Autodesk Inventor part; units mm, degrees
ref_plane "YZ Plane" through (0, 0, 0) normal (1, 0, 0) x (0, 1, 0)
ref_plane "XZ Plane" through (0, 0, 0) normal (0, 1, 0) x (-1, 0, 0)
ref_plane "XY Plane" through (0, 0, 0) normal (0, 0, 1) x (1, 0, 0)
sketch "Skizze1" plane through (0, 0, 0) normal (0, 0, 1) x (1, 0, 0)
  circle A0 centre (0, 0) radius 11
  dimension "d0" = 22
extrude "Extrusion1" add sketch "Skizze1" along normal blind 50.5
sketch "Skizze2" plane through (0, 0, 50.5) normal (0, 0, 1) x (1, 0, 0)
  circle A0 centre (0, 0) radius 3
  circle A1 centre (0, 0) radius 2.5
  circle A2 centre (0, 0) radius 1.5
  dimension "d3" = 6
  dimension "d4" = 5
  dimension "d9" = 3
extrude "Extrusion2" add sketch "Skizze2" along normal blind 1 contours A0 | A1 | A2
extrude "Extrusion3" add sketch "Skizze2" along normal blind 2.5 contours A1 | A2
extrude "Extrusion4" add sketch "Skizze2" along normal blind 11.5 contours A2
properties part number "MotorStanger"
Geometry: final body of the model. Coordinates: model frame, mm. A direction names the side the tool comes from. Round coordinates to 2 decimals unless told otherwise and drop trailing zeros. Order: outer loops, then holes, each group sorted by start corner. A loop starts at its lowest first (then second) coordinate and runs counter-clockwise, first axis right, second up.
Q1. Section C-C, the plane z = 23.5. Output: boundary loops of the cut face in (x, y), and give its area (3 significant figures).
Result sheet:
outline: circle Ø22 at (0, 0)
area: 380 mm2
Q2. Material intervals for probe 1 along Z at (x, y) = (-6, 6.5); probe 2 along Y at (x, z) = (-0.25, 14.5); probe 3 along X at (y, z) = (2.75, 48), sorted ascending.
Result sheet:
probe 1: z = 0 to 50.5
probe 2: y = -11 to 11
probe 3: x = -10.65 to 10.65
Q3. Access query for faces 1 (the face through (-2.38, 10.74, 24.9)), 2 (the face through (-0.54, 2.44, 52.24)). Directions: +Z, -Z, +X, -X, +Y, -Y. A direction counts if a zero-diameter tool reaches every point of the face in a straight line with its end or side. Return the directions, or none.
Result sheet:
face 1: +Z, -Z
face 2: +Z
Q4. Pin query (flat end, axial travel): pin 1 (12 mm diameter, centred on x = 2, y = -7.5, fed in from +Z); pin 2 (2 mm diameter, centred on x = -8, z = 17, fed in from -Y); pin 3 (2 mm diameter, centred on y = 3, z = 21, fed in from -X). Return the tip coordinate at first contact, or that it passes through.
Result sheet:
pin 1: stops at z = 53
pin 2: stops at y = -8.49
pin 3: stops at x = -10.82
Q5. Section A-A, the plane x = 0. Output: boundary loops of the cut face in (y, z).
Result sheet:
outline: (-11, 0) - (11, 0) - (11, 50.5) - (3, 50.5) - (3, 51.5) - (2.5, 51.5) - (2.5, 53) - (1.5, 53) - (1.5, 62) - (-1.5, 62) - (-1.5, 53) - (-2.5, 53) - (-2.5, 51.5) - (-3, 51.5) - (-3, 50.5) - (-11, 50.5) - close
Q6. Section D-D, the plane y = 7.5. Output: boundary loops of the cut face in (x, z), and give its area (3 significant figures).
Result sheet:
outline: (-8.05, 0) - (8.05, 0) - (8.05, 50.5) - (-8.05, 50.5) - close
area: 813 mm2
